Read the model definition and answer for the solid it produces. Units are mm, in the model's axes. A direction names the side the tool comes from. Coordinates: 2 decimals unless noted, no trailing zeros. Write each loop counter-clockwise with the first axis right and the second up, starting at its lowest first coordinate (ties: lowest second). Pieces come first, ordered by that corner, then holes. Notation, with made-up numbers: (52.25, 87) -> (74.25, 87) arc R13 ccw to (74.25, 97) -> close; hole circle Ø6 at (-16.75, -10.75). An arc over 180 degrees is marked (long way). Answer in a Markdown table with one row per item. Add a question column.
Item 1: Section B-B on y = 1.2 is taken. Write down the section's boundary in (x, z), then the cut area to 3 significant figures.
Item 2: Straight lines are drawn through the part: line 1 (X direction, y = 2.3, z = 0); line 2 (Y direction, x = 13, z = -6); line 3 (Z direction, x = 4, y = 1.1). For each, find the intervals that lie inside material, in ascending order. Write a range as from..to.
Item 3: For a pull along X with two mould halves and no side action, classify faces 1 (the face through (3.648, 2.308, -3.978)), 2 (the face through (3, 3.81, -1)), 3 (the face through (-0.9, 1.88, -2.86)) as +X half, -X half, draft (parallel to the pull), parting line (faces both ways), or undercut.
Item 4: Given pin 1 Ø3 at (x, z) = (-7.5, 8.5) entering from +Y; pin 2 Ø8 at (x, z) = (0, 0) entering from +Y; pin 3 Ø2 at (y, z) = (1.5, -11) entering from +X; pin 4 Ø1 at (x, y) = (-6, 1) entering from +Z, each flat-ended and moving along its own axis, determine where each tip first touches the part or whether it passes through.
Item 5: Which of the six approach directions +Z, -Z, +X, -X, +Y, -Y give full straight-line access (tool end or side, diameter ignored) to faces 4 (the face through (-0.21, 0, -3.15)), 5 (the face through (0, 1.588, -7))?
```python
from build123d import *

# Parameters (mm, degrees)
SKETCH1_R           = 15.875
SKETCH1_R_2         = 3
BOSS_EXTRUDE1_DEPTH = 3.81
CUT_EXTRUDE1_START  = -2.2225
SKETCH2_R           = 15.875
SKETCH2_R_2         = 5.3975
CUT_EXTRUDE1_DEPTH  = 2.2225
FILLET1_R           = 0.762


with BuildPart() as part:
    # Sketch1 → Boss-Extrude1 (new body)
    with BuildSketch(Plane(origin=(0, 0, 0), x_dir=(1, 0, 0), z_dir=(0, 1, 0))):
        with Locations(Location((0, 0, 0), (0, 0, 90))):
            Circle(SKETCH1_R)
        with Locations(Location((0, 0, 0), (0, 0, 90))):
            Circle(SKETCH1_R_2, mode=Mode.SUBTRACT)
    extrude(amount=BOSS_EXTRUDE1_DEPTH)

    # Sketch2 → Cut-Extrude1 (cut)
    with BuildSketch(Plane(origin=(0, 3.81, 0), x_dir=(1, 0, 0), z_dir=(0, 1, 0)).offset(CUT_EXTRUDE1_START)):
        with Locations(Location((0, 0, 0), (0, 0, 90))):
            Circle(SKETCH2_R)
        with Locations(Location((0, 0, 0), (0, 0, 270))):
            Circle(SKETCH2_R_2, mode=Mode.SUBTRACT)
    extrude(amount=CUT_EXTRUDE1_DEPTH, mode=Mode.SUBTRACT)

    # Fillet1
    fillet1_edges = [part.edges().sort_by_distance(p)[0] for p in [
        (0, 3.81, -5.3975),
        (0, 1.5875, 15.875),
        (0, 0, 15.875),
    ]]
    fillet(fillet1_edges, radius=FILLET1_R)


solid = part.part
```
Results below:
| question | item | result |
|---|---|---|
| 1 | outline | circle Ø31.55 at (0, 0); hole circle Ø6 at (0, 0) |
| 1 | area | 754 mm2 |
| 2 | line 1 | x = -5.4..-3, 3..5.4 |
| 2 | line 2 | y = 0..1.59 |
| 2 | line 3 | z = -15.31..15.31 |
| 3 | face 1 | parting line |
| 3 | face 2 | draft |
| 3 | face 3 | undercut |
| 4 | pin 1 | stops at y = 1.59 |
| 4 | pin 2 | stops at y = 3.81 |
| 4 | pin 3 | stops at x = 12.2 |
| 4 | pin 4 | stops at z = 14.88 |
| 5 | face 4 | +Z, -Z, +X, -X, -Y |
| 5 | face 5 | +Y |
